```python
from build123d import *

# Parameters (mm, degrees)
RESSALTO_EXTRUS_O1_DEPTH      = 2.5
ESBO_O2_R                     = 5.5
CORTE_EXTRUS_O1_DEPTH         = 5
ESBO_O3_R                     = 1.25
CORTE_EXTRUS_O2_DEPTH         = 5
PADR_OCIRCULAR1_COUNT         = 8
ESPELHAR1_COPY_1_SKETCH_R     = 1.25
ESPELHAR1_COPY_1_DEPTH        = 5
ESPELHAR1_COPY_2_SKETCH_R     = 1.25
ESPELHAR1_COPY_2_DEPTH        = 5
ESPELHAR1_COPY_3_SKETCH_R     = 1.25
ESPELHAR1_COPY_3_DEPTH        = 5
ESPELHAR1_COPY_4_SKETCH_R     = 1.25
ESPELHAR1_COPY_4_DEPTH        = 5
ESPELHAR1_COPY_5_SKETCH_R     = 1.25
ESPELHAR1_COPY_5_DEPTH        = 5
ESPELHAR1_COPY_6_SKETCH_R     = 1.25
ESPELHAR1_COPY_6_DEPTH        = 5
ESPELHAR1_COPY_7_SKETCH_R     = 1.25
ESPELHAR1_COPY_7_DEPTH        = 5
CORTE_EXTRUS_O5_DEPTH         = 74.078475416
CORTE_EXTRUS_O5_DEPTH_BACK    = 74.078475416
CONVERTER_S_LIDO1_START       = -2.5
CONVERTER_S_LIDO1_OUTLINE_R   = 1.25
CONVERTER_S_LIDO1_OUTLINE_R_2 = 5.5
CONVERTER_S_LIDO1_DEPTH       = 3
ESBO_O8_R                     = 1.5
CORTE_EXTRUS_O3_DEPTH         = 2
PADR_O_LINEAR1_COUNT          = 7
PADR_O_LINEAR1_PITCH          = 10
CORTE_EXTRUS_O4_DEPTH         = 2


# Read off the part's stored shape, not the designer's step: Converter-Sólido1
with BuildPart() as part:
    # Esboço1 → Ressalto-extrusão1 (new, symmetric)
    with BuildSketch(Plane.XY):
        with BuildLine():
            Line((-59.430402553, 19.151096923), (62.502392295, 19.151096923))
            ThreePointArc((62.502392295, 19.151096923), (69.19383205, 18.276167196), (65.569597447, 12.583558694))
            Line((65.569597447, 12.583558694), (65.569597447, -13.806757673))
            ThreePointArc((65.569597447, -13.806757673), (69.322501763, -19.190849142), (62.972416023, -20.848903077))
            Line((62.972416023, -20.848903077), (-59.430402553, -20.848903077))
            Line((-59.430402553, -20.848903077), (-59.430402553, 19.151096923))
        make_face()
    extrude(amount=RESSALTO_EXTRUS_O1_DEPTH, both=True)

    # Esboço2 → Corte-extrusão1 (cut)
    with BuildSketch(Plane.XY.offset(2.5)):
        with Locations((-44.430402553, 0)):
            Circle(ESBO_O2_R)
    corte_extrus_o1 = extrude(amount=-CORTE_EXTRUS_O1_DEPTH, mode=Mode.SUBTRACT)

    # Esboço3 → Corte-extrusão2 (cut)
    with BuildSketch(Plane.XY.offset(2.5)):
        with Locations((-55.430402553, 0)):
            Circle(ESBO_O3_R)
    corte_extrus_o2 = extrude(amount=-CORTE_EXTRUS_O2_DEPTH, mode=Mode.SUBTRACT)

    # PadrãoCircular1: Corte-extrusão2 ×8 about axis
    padr_ocircular1_axis = Axis((-44.430402553, 0, 0), (0, 0, 1))
    for i in range(1, PADR_OCIRCULAR1_COUNT):
        add(corte_extrus_o2.rotate(padr_ocircular1_axis, i * 360 / PADR_OCIRCULAR1_COUNT), mode=Mode.SUBTRACT)

    # Espelhar1: Corte-extrusão1, Corte-extrusão2 across plane
    add(corte_extrus_o1.mirror(Plane(origin=(0, 0, 0), x_dir=(0, 0, 1), z_dir=(1, 0, 0))), mode=Mode.SUBTRACT)
    add(corte_extrus_o2.mirror(Plane(origin=(0, 0, 0), x_dir=(0, 0, 1), z_dir=(1, 0, 0))), mode=Mode.SUBTRACT)

    # Espelhar1 copy 1 sketch → Espelhar1 copy 1 (cut)
    with BuildSketch(Plane(origin=(13.013363617, 31.417038936, 2.5), x_dir=(-0.7071067811865476, 0.7071067811865475, 0), z_dir=(0, 0, 1))):
        with Locations((-55.430402553, 0)):
            Circle(ESPELHAR1_COPY_1_SKETCH_R)
    extrude(amount=-ESPELHAR1_COPY_1_DEPTH, mode=Mode.SUBTRACT)

    # Espelhar1 copy 2 sketch → Espelhar1 copy 2 (cut)
    with BuildSketch(Plane(origin=(44.430402553, 44.430402553, 2.5), x_dir=(0, 1, 0), z_dir=(0, 0, 1))):
        with Locations((-55.430402553, 0)):
            Circle(ESPELHAR1_COPY_2_SKETCH_R)
    extrude(amount=-ESPELHAR1_COPY_2_DEPTH, mode=Mode.SUBTRACT)

    # Espelhar1 copy 3 sketch → Espelhar1 copy 3 (cut)
    with BuildSketch(Plane(origin=(75.847441489, 31.417038936, 2.5), x_dir=(0.7071067811865475, 0.7071067811865476, 0), z_dir=(0, 0, 1))):
        with Locations((-55.430402553, 0)):
            Circle(ESPELHAR1_COPY_3_SKETCH_R)
    extrude(amount=-ESPELHAR1_COPY_3_DEPTH, mode=Mode.SUBTRACT)

    # Espelhar1 copy 4 sketch → Espelhar1 copy 4 (cut)
    with BuildSketch(Plane(origin=(88.860805106, 0, 2.5), x_dir=(1, 0, 0), z_dir=(0, 0, 1))):
        with Locations((-55.430402553, 0)):
            Circle(ESPELHAR1_COPY_4_SKETCH_R)
    extrude(amount=-ESPELHAR1_COPY_4_DEPTH, mode=Mode.SUBTRACT)

    # Espelhar1 copy 5 sketch → Espelhar1 copy 5 (cut)
    with BuildSketch(Plane(origin=(75.847441489, -31.417038936, 2.5), x_dir=(0.7071067811865477, -0.7071067811865475, 0), z_dir=(0, 0, 1))):
        with Locations((-55.430402553, 0)):
            Circle(ESPELHAR1_COPY_5_SKETCH_R)
    extrude(amount=-ESPELHAR1_COPY_5_DEPTH, mode=Mode.SUBTRACT)

    # Espelhar1 copy 6 sketch → Espelhar1 copy 6 (cut)
    with BuildSketch(Plane(origin=(44.430402553, -44.430402553, 2.5), x_dir=(0, -1, 0), z_dir=(0, 0, 1))):
        with Locations((-55.430402553, 0)):
            Circle(ESPELHAR1_COPY_6_SKETCH_R)
    extrude(amount=-ESPELHAR1_COPY_6_DEPTH, mode=Mode.SUBTRACT)

    # Espelhar1 copy 7 sketch → Espelhar1 copy 7 (cut)
    with BuildSketch(Plane(origin=(13.013363617, -31.417038936, 2.5), x_dir=(-0.7071067811865474, -0.7071067811865477, 0), z_dir=(0, 0, 1))):
        with Locations((-55.430402553, 0)):
            Circle(ESPELHAR1_COPY_7_SKETCH_R)
    extrude(amount=-ESPELHAR1_COPY_7_DEPTH, mode=Mode.SUBTRACT)

    # Esboço10 → Corte-extrusão5 (cut, two sides: drawn at the far end of the back side and taken through both)
    with BuildSketch(Plane(origin=(0, 0, -2.5), x_dir=(-1, 0, 0), z_dir=(0, 0, -1)).offset(-CORTE_EXTRUS_O5_DEPTH_BACK)):
        with BuildLine():
            Line((50.985622588, 13.491815678), (39.337809239, 19.151096923))
            Line((39.337809239, 19.151096923), (39.337809239, 27.419939303))
            Line((39.337809239, 27.419939303), (72.861321118, 27.419939303))
            Line((72.861321118, 27.419939303), (72.861321118, -27.215460657))
            Line((72.861321118, -27.215460657), (25.772247119, -27.215460657))
            Line((25.772247119, -27.215460657), (25.772247119, -20.848903077))
            Line((25.772247119, -20.848903077), (52.073972286, -12.906426373))
            ThreePointArc((52.073972286, -12.906426373), (59.417670602, 0.617896776), (50.985622588, 13.491815678))
        make_face()
    extrude(amount=CORTE_EXTRUS_O5_DEPTH + CORTE_EXTRUS_O5_DEPTH_BACK, mode=Mode.SUBTRACT)

    # Converter-Sólido1 outline → Converter-Sólido1 (cut)
    with BuildSketch(Plane.XY.offset(CONVERTER_S_LIDO1_START)):
        with BuildLine():
            Line((62.502392295, 19.151096923), (-39.337809239, 19.151096923))
            Line((-39.337809239, 19.151096923), (-50.985622588, 13.491815678))
            ThreePointArc((-50.985622588, 13.491815678), (-59.417670602, 0.617896776), (-52.073972286, -12.906426373))
            Line((-52.073972286, -12.906426373), (-25.772247119, -20.848903077))
            Line((-25.772247119, -20.848903077), (62.972416023, -20.848903077))
            ThreePointArc((62.972416023, -20.848903077), (69.322501763, -19.190849142), (65.569597447, -13.806757673))
            Line((65.569597447, -13.806757673), (65.569597447, 12.583558694))
            ThreePointArc((65.569597447, 12.583558694), (69.19383205, 18.276167196), (62.502392295, 19.151096923))
        make_face()
        with Locations((-44.430402553, -11)):
            Circle(CONVERTER_S_LIDO1_OUTLINE_R, mode=Mode.SUBTRACT)
        with Locations((-52.208577146, -7.778174593)):
            Circle(CONVERTER_S_LIDO1_OUTLINE_R, mode=Mode.SUBTRACT)
        with Locations((-36.65222796, -7.778174593)):
            Circle(CONVERTER_S_LIDO1_OUTLINE_R, mode=Mode.SUBTRACT)
        with Locations((36.65222796, -7.778174593)):
            Circle(CONVERTER_S_LIDO1_OUTLINE_R, mode=Mode.SUBTRACT)
        with Locations((44.430402553, -11)):
            Circle(CONVERTER_S_LIDO1_OUTLINE_R, mode=Mode.SUBTRACT)
        with Locations((52.208577146, -7.778174593)):
            Circle(CONVERTER_S_LIDO1_OUTLINE_R, mode=Mode.SUBTRACT)
        with Locations((-55.430402553, 0)):
            Circle(CONVERTER_S_LIDO1_OUTLINE_R, mode=Mode.SUBTRACT)
        with Locations((-44.430402553, 0)):
            Circle(CONVERTER_S_LIDO1_OUTLINE_R_2, mode=Mode.SUBTRACT)
        with Locations((-33.430402553, 0)):
            Circle(CONVERTER_S_LIDO1_OUTLINE_R, mode=Mode.SUBTRACT)
        with Locations((-52.208577146, 7.778174593)):
            Circle(CONVERTER_S_LIDO1_OUTLINE_R, mode=Mode.SUBTRACT)
        with Locations((-36.65222796, 7.778174593)):
            Circle(CONVERTER_S_LIDO1_OUTLINE_R, mode=Mode.SUBTRACT)
        with Locations((-44.430402553, 11)):
            Circle(CONVERTER_S_LIDO1_OUTLINE_R, mode=Mode.SUBTRACT)
        with Locations((33.430402553, 0)):
            Circle(CONVERTER_S_LIDO1_OUTLINE_R, mode=Mode.SUBTRACT)
        with Locations((36.65222796, 7.778174593)):
            Circle(CONVERTER_S_LIDO1_OUTLINE_R, mode=Mode.SUBTRACT)
        with Locations((44.430402553, 0)):
            Circle(CONVERTER_S_LIDO1_OUTLINE_R_2, mode=Mode.SUBTRACT)
        with Locations((55.430402553, 0)):
            Circle(CONVERTER_S_LIDO1_OUTLINE_R, mode=Mode.SUBTRACT)
        with Locations((52.208577146, 7.778174593)):
            Circle(CONVERTER_S_LIDO1_OUTLINE_R, mode=Mode.SUBTRACT)
        with Locations((44.430402553, 11)):
            Circle(CONVERTER_S_LIDO1_OUTLINE_R, mode=Mode.SUBTRACT)
    extrude(amount=CONVERTER_S_LIDO1_DEPTH, mode=Mode.SUBTRACT)

    # Esboço8 → Corte-extrusão3 (cut)
    with BuildSketch(Plane(origin=(0, 0, 0.5), x_dir=(-1, 0, 0), z_dir=(0, 0, -1))):
        with Locations((26.430402553, 16.151096923)):
            Circle(ESBO_O8_R)
        with Locations((26.430402553, -17.848903077)):
            Circle(ESBO_O8_R)
    corte_extrus_o3 = extrude(amount=-CORTE_EXTRUS_O3_DEPTH, mode=Mode.SUBTRACT)

    # Padrão linear1: Corte-extrusão3 ×7
    with Locations(*[(i * PADR_O_LINEAR1_PITCH, 0, 0) for i in range(1, PADR_O_LINEAR1_COUNT)]):
        add(corte_extrus_o3, mode=Mode.SUBTRACT)

    # Esboço9 → Corte-extrusão4 (cut)
    with BuildSketch(Plane(origin=(0, 0, 0.5), x_dir=(-1, 0, 0), z_dir=(0, 0, -1))):
        with BuildLine():
            Line((-22.912822242, 5.229141159), (22.912822242, 5.229141159))
            ThreePointArc((22.912822242, 5.229141159), (28.1419634, 0), (22.912822242, -5.229141159))
            Line((22.912822242, -5.229141159), (-22.912822242, -5.229141159))
            ThreePointArc((-22.912822242, -5.229141159), (-28.1419634, 0), (-22.912822242, 5.229141159))
        make_face()
    extrude(amount=-CORTE_EXTRUS_O4_DEPTH, mode=Mode.SUBTRACT)


solid = part.part
```
Input: part model. Units: mm. Frame: model coordinates. A direction names the side the tool comes from. Give positions to 0.01 mm unless a question says otherwise; leave off trailing zeros. Order: outer loops, then holes, each group sorted by start corner. A loop starts at its lowest first (then second) coordinate and runs counter-clockwise, first axis right, second up.
1. Pin query (flat end, axial travel): pin 1 Ø1 at (x, z) = (1, 1.5) entering from -Y; pin 2 Ø1.8 at (x, y) = (-26.43, -17.85) entering from +Z; pin 3 Ø1 at (y, z) = (1.5, 1.5) entering from -X; pin 4 Ø5 at (x, y) = (23.57, 16.15) entering from -Z. Return the tip coordinate at first contact, or that it passes through.
Computed:
pin 1: stops at y = -20.85
pin 2: passes through
pin 3: stops at x = -59.4
pin 4: stops at z = 0.5
2. Cut plane B-B (y = 0). State how many separate pieces and enclosed holes the cut face has, and give its area (3 significant figures).
Computed:
separate pieces: 8
enclosed holes: 0
area: 73.4 mm2
3. Cut plane C-C (y = 11). Return loops of the section in (x, z).
Computed:
outline: (-54.63, 0.5) - (-45.68, 0.5) - (-45.68, 2.5) - (-54.63, 2.5) - close; (-43.18, 0.5) - (43.18, 0.5) - (43.18, 2.5) - (-43.18, 2.5) - close; (45.68, 0.5) - (65.57, 0.5) - (65.57, 2.5) - (45.68, 2.5) - close
4. Cut plane D-D (x = 26.5). Return loops of the section in (y, z).
Computed:
outline: (-20.85, 0.5) - (-3.8, 0.5) - (-3.8, 2.5) - (-20.85, 2.5) - close; (3.8, 0.5) - (19.15, 0.5) - (19.15, 2.5) - (3.8, 2.5) - close
5. Draft query along Y for faces 3 (the face through (4, 9, 0.5)), 4 (the face through (-51.054, -7.3, 1.514)), 5 (the face through (-45.243, 16.282, 1.514)), 6 (the face through (-14.93, -17.78, 1.49)). Return one class per face: released by +Y, released by -Y, zero draft, split by the parting line, or undercut.
Computed:
face 3: zero draft
face 4: undercut
face 5: released by +Y
face 6: undercut
6. Set-up query: faces 1 (the face through (-28.14, 0.11, 1.49)), 2 (the face through (-38.739, -16.933, 1.514)). Return all of +Z, -Z, +X, -X, +Y, -Y with unobstructed straight access to the full face (end or side cutting, diameter ignored); none if empty.
Computed:
face 1: +Z, -Z
face 2: +Z, -Z, -X, -Y
7. Cut plane A-A (x = 10). Return loops of the section in (y, z).
Computed:
outline: (-20.85, 0.5) - (-5.23, 0.5) - (-5.23, 2.5) - (-20.85, 2.5) - close; (5.23, 0.5) - (19.15, 0.5) - (19.15, 2.5) - (5.23, 2.5) - close
8. Line query: probe 1 along Y at (x, z) = (-21, 0.85); probe 2 along Y at (x, z) = (-27, 0.8); probe 3 along Y at (x, z) = (37.5, 0.85). Output: solid intervals per line, ascending.
Computed:
probe 1: y = -20.85 to -5.23, 5.23 to 19.15
probe 2: y = -20.48 to -19.24, -16.46 to -3.26, 3.26 to 14.76, 17.54 to 19.15
probe 3: y = -20.85 to -8.7, -6.86 to 6.86, 8.7 to 19.15
